Could you check a few things on this model? Use its own coordinates, in mm. A direction names the side the tool comes from. Give positions to 0.01 mm unless a question says otherwise; leave off trailing zeros. Write each loop counter-clockwise with the first axis right and the second up, starting at its lowest first coordinate (ties: lowest second). Pieces come first, ordered by that corner, then holes. Notation, with made-up numbers: M 59.5,16 L 107.5,16 A30 cw 107.5,53 Z; hole C -38.75,64.5 d5. An arc over 180 degrees is marked long. Write each question's results on one line, items separated by ' | '. Start each with the question number.
from build123d import *

# Parameters (mm, degrees)
S_CYL1_R        = 19
BOSS_1_DEPTH    = 7
BOSS_2_DEPTH    = 2.1
S_BOX3_W        = 28.2
S_BOX3_H        = 10
BOSS_3_DEPTH    = 1.5
S_BOX4_W        = 37.6
S_BOX4_H        = 47
BOSS_4_DEPTH    = 14.2
BOSS_5_DEPTH    = 23
BOSS_6_DEPTH    = 22
S_BOX7_W        = 36.1
S_BOX7_H        = 3
BOSS_7_DEPTH    = 31.8
S_BOX8_W        = 36.1
S_BOX8_H        = 3
BOSS_8_DEPTH    = 31.8
S_BOX9_W        = 36.1
S_BOX9_H        = 52.4
BOSS_9_DEPTH    = 3
S_BOX10_W       = 36.1
S_BOX10_H       = 52.4
BOSS_10_DEPTH   = 3
S_BOX11_W       = 4.6
S_BOX11_H       = 52.4
BOSS_11_DEPTH   = 31.8
S_HOLE12_R      = 10.5
HOLE_12_DEPTH   = 4.8
S_CUT13_W       = 4.75
S_CUT13_H       = 19.5
POCKET_13_DEPTH = 19.4
S_CUT14_W       = 4.75
S_CUT14_H       = 8.8
POCKET_14_DEPTH = 16.4
S_CUT15_W       = 4.75
S_CUT15_H       = 11
POCKET_15_DEPTH = 7
S_CUT16_W       = 2.9
S_CUT16_H       = 20
POCKET_16_DEPTH = 16.4
S_HOLE17_R      = 1.1
HOLE_17_DEPTH   = 4.8
S_HOLE18_R      = 2.3
HOLE_18_DEPTH   = 1.7
S_HOLE19_R      = 1.1
HOLE_19_DEPTH   = 4.8
S_HOLE20_R      = 2.3
HOLE_20_DEPTH   = 1.7
S_HOLE21_R      = 1.1
HOLE_21_DEPTH   = 4.8
S_HOLE22_R      = 2.3
HOLE_22_DEPTH   = 1.7
CUT_23_DEPTH    = 6.1
S_HOLE24_R      = 3.5
HOLE_24_DEPTH   = 10.6
S_HOLE25_R      = 1.7
HOLE_25_DEPTH   = 10.6
S_HOLE26_R      = 1.7
HOLE_26_DEPTH   = 10.6
S_HOLE27_R      = 1.7
HOLE_27_DEPTH   = 10.6
S_HOLE28_R      = 1.7
HOLE_28_DEPTH   = 10.6
S_HOLE29_R      = 3.2
HOLE_29_DEPTH   = 7.6
S_HOLE30_R      = 3.2
HOLE_30_DEPTH   = 7.6
S_HOLE31_R      = 3.2
HOLE_31_DEPTH   = 7.6
S_HOLE32_R      = 3.2
HOLE_32_DEPTH   = 7.6


with BuildPart() as part:
    # S_cyl1 → Boss_1 (new body)
    with BuildSketch(Plane.XY.offset(23)):
        Circle(S_CYL1_R)
    extrude(amount=BOSS_1_DEPTH)

    # S_prism2 → Boss_2 (add)
    with BuildSketch(Plane.XY.offset(21)):
        with BuildLine():
            Line((-15.491933385, -11), (15.491933385, -11))
            ThreePointArc((15.491933385, -11), (19, 0), (15.491933385, 11))
            Line((15.491933385, 11), (-15.491933385, 11))
            ThreePointArc((-15.491933385, 11), (-19, 0), (-15.491933385, -11))
        make_face()
    extrude(amount=BOSS_2_DEPTH)

    # S_box3 → Boss_3 (add)
    with BuildSketch(Plane.XY.offset(19.6)):
        with Locations((-0.1, 0)):
            Rectangle(S_BOX3_W, S_BOX3_H)
    extrude(amount=BOSS_3_DEPTH)

    # S_box4 → Boss_4 (add)
    with BuildSketch(Plane.XY.offset(15.8)):
        with Locations((-35.2, -11.5)):
            Rectangle(S_BOX4_W, S_BOX4_H)
    extrude(amount=BOSS_4_DEPTH)

    # S_prism5 → Boss_5 (add)
    with BuildSketch(Plane(origin=(-11.5, 0, 0), x_dir=(0, 0, -1), z_dir=(1, 0, 0))):
        Polygon((-21.05, -11), (-21.05, 12), (-23.1, 15), (-23.1, -12.5), align=None)
    extrude(amount=BOSS_5_DEPTH)

    # S_prism6 → Boss_6 (add)
    with BuildSketch(Plane(origin=(0, -11, 0), x_dir=(1, 0, 0), z_dir=(0, 1, 0))):
        Polygon((-16.45, -21.1), (-16.45, -19.9), (-14.8, -21.1), align=None)
    extrude(amount=BOSS_6_DEPTH)

    # S_box8 → Boss_8 (add)
    with BuildSketch(Plane.XY.offset(-15.9)):
        with Locations((-36.85, 12.2)):
            Rectangle(S_BOX8_W, S_BOX8_H)
    extrude(amount=BOSS_8_DEPTH)



with BuildPart() as body_2:
    # S_box7 → Boss_7 (new body)
    with BuildSketch(Plane.XY.offset(-15.9)):
        with Locations((-36.85, -37.2)):
            Rectangle(S_BOX7_W, S_BOX7_H)
    extrude(amount=BOSS_7_DEPTH)


with BuildPart() as part_1:
    add(part.part)

    add(body_2.part)  # Boss_9 merges body 2
    # S_box9 → Boss_9 (add)
    with BuildSketch(Plane.XY.offset(-15.9)):
        with Locations((-36.85, -12.5)):
            Rectangle(S_BOX9_W, S_BOX9_H)
    extrude(amount=BOSS_9_DEPTH)

    # S_box10 → Boss_10 (add)
    with BuildSketch(Plane.XY.offset(12.9)):
        with Locations((-36.85, -12.5)):
            Rectangle(S_BOX10_W, S_BOX10_H)
    extrude(amount=BOSS_10_DEPTH)

    # S_box11 → Boss_11 (add)
    with BuildSketch(Plane.XY.offset(-15.9)):
        with Locations((-52.6, -12.5)):
            Rectangle(S_BOX11_W, S_BOX11_H)
    extrude(amount=BOSS_11_DEPTH)

    # S_hole12 → Hole_12 (cut)
    with BuildSketch(Plane(origin=(-55, 0, 0), x_dir=(0, 0, -1), z_dir=(1, 0, 0))):
        with Locations(Location((0, 0, 0), (0, 0, 180))):
            Circle(S_HOLE12_R)
    extrude(amount=HOLE_12_DEPTH, mode=Mode.SUBTRACT)

    # S_cut13 → Pocket_13 (cut)
    with BuildSketch(Plane.XY.offset(-9.7)):
        with Locations((-52.625, -20.65)):
            Rectangle(S_CUT13_W, S_CUT13_H)
    extrude(amount=POCKET_13_DEPTH, mode=Mode.SUBTRACT)

    # S_cut14 → Pocket_14 (cut)
    with BuildSketch(Plane.XY.offset(-8.2)):
        with Locations((-52.625, -34.8)):
            Rectangle(S_CUT14_W, S_CUT14_H)
    extrude(amount=POCKET_14_DEPTH, mode=Mode.SUBTRACT)

    # S_cut15 → Pocket_15 (cut)
    with BuildSketch(Plane.XY.offset(-3.5)):
        with Locations((-52.625, -5.5)):
            Rectangle(S_CUT15_W, S_CUT15_H)
    extrude(amount=POCKET_15_DEPTH, mode=Mode.SUBTRACT)

    # S_cut16 → Pocket_16 (cut)
    with BuildSketch(Plane.XY.offset(-16.4)):
        with Locations((-53.65, 0)):
            Rectangle(S_CUT16_W, S_CUT16_H)
    extrude(amount=POCKET_16_DEPTH, mode=Mode.SUBTRACT)

    # S_hole17 → Hole_17 (cut)
    with BuildSketch(Plane(origin=(-55, 0, 0), x_dir=(0, 0, -1), z_dir=(1, 0, 0))):
        with Locations(Location((-10.25, -8.3, 0), (0, 0, 180))):
            Circle(S_HOLE17_R)
    extrude(amount=HOLE_17_DEPTH, mode=Mode.SUBTRACT)

    # S_hole18 → Hole_18 (cut)
    with BuildSketch(Plane(origin=(-55, 0, 0), x_dir=(0, 0, -1), z_dir=(1, 0, 0))):
        with Locations((-10.25, -8.3)):
            Circle(S_HOLE18_R)
    extrude(amount=HOLE_18_DEPTH, mode=Mode.SUBTRACT)

    # S_hole19 → Hole_19 (cut)
    with BuildSketch(Plane(origin=(-55, 0, 0), x_dir=(0, 0, -1), z_dir=(1, 0, 0))):
        with Locations(Location((10.25, -32.75, 0), (0, 0, 180))):
            Circle(S_HOLE19_R)
    extrude(amount=HOLE_19_DEPTH, mode=Mode.SUBTRACT)

    # S_hole20 → Hole_20 (cut)
    with BuildSketch(Plane(origin=(-55, 0, 0), x_dir=(0, 0, -1), z_dir=(1, 0, 0))):
        with Locations((10.25, -32.75)):
            Circle(S_HOLE20_R)
    extrude(amount=HOLE_20_DEPTH, mode=Mode.SUBTRACT)

    # S_hole21 → Hole_21 (cut)
    with BuildSketch(Plane(origin=(-55, 0, 0), x_dir=(0, 0, -1), z_dir=(1, 0, 0))):
        with Locations(Location((-10.25, -32.75, 0), (0, 0, 180))):
            Circle(S_HOLE21_R)
    extrude(amount=HOLE_21_DEPTH, mode=Mode.SUBTRACT)

    # S_hole22 → Hole_22 (cut)
    with BuildSketch(Plane(origin=(-55, 0, 0), x_dir=(0, 0, -1), z_dir=(1, 0, 0))):
        with Locations((-10.25, -32.75)):
            Circle(S_HOLE22_R)
    extrude(amount=HOLE_22_DEPTH, mode=Mode.SUBTRACT)

    # S_pcut23 → Cut_23 (cut)
    with BuildSketch(Plane.XY.offset(20.9)):
        with BuildLine():
            Line((-14.792307772, 12.858756968), (-11.547056577, 10.037703144))
            ThreePointArc((-11.547056577, 10.037703144), (11.72047998, 9.834650428), (7.880082546, -13.114659701))
            Line((7.880082546, -13.114659701), (10.094746268, -16.800479094))
            ThreePointArc((10.094746268, -16.800479094), (15.014471085, 12.59863715), (-14.792307772, 12.858756968))
        make_face()
    extrude(amount=CUT_23_DEPTH, mode=Mode.SUBTRACT)

    # S_hole24 → Hole_24 (cut)
    with BuildSketch(Plane.XY.offset(19.5)):
        Circle(S_HOLE24_R)
    extrude(amount=HOLE_24_DEPTH, mode=Mode.SUBTRACT)

    # S_hole25 → Hole_25 (cut)
    with BuildSketch(Plane.XY.offset(19.5)):
        with Locations((7, 0)):
            Circle(S_HOLE25_R)
    extrude(amount=HOLE_25_DEPTH, mode=Mode.SUBTRACT)

    # S_hole26 → Hole_26 (cut)
    with BuildSketch(Plane.XY.offset(19.5)):
        with Locations((0, 7)):
            Circle(S_HOLE26_R)
    extrude(amount=HOLE_26_DEPTH, mode=Mode.SUBTRACT)

    # S_hole27 → Hole_27 (cut)
    with BuildSketch(Plane.XY.offset(19.5)):
        with Locations((-7, 0)):
            Circle(S_HOLE27_R)
    extrude(amount=HOLE_27_DEPTH, mode=Mode.SUBTRACT)

    # S_hole28 → Hole_28 (cut)
    with BuildSketch(Plane.XY.offset(19.5)):
        with Locations((0, -7)):
            Circle(S_HOLE28_R)
    extrude(amount=HOLE_28_DEPTH, mode=Mode.SUBTRACT)

    # S_hole29 → Hole_29 (cut)
    with BuildSketch(Plane.XY.offset(19.4)):
        with Locations(Location((7, 0, 0), (0, 0, 180))):
            Circle(S_HOLE29_R)
    extrude(amount=HOLE_29_DEPTH, mode=Mode.SUBTRACT)

    # S_hole30 → Hole_30 (cut)
    with BuildSketch(Plane.XY.offset(19.4)):
        with Locations(Location((0, 7, 0), (0, 0, 218.682187453))):
            Circle(S_HOLE30_R)
    extrude(amount=HOLE_30_DEPTH, mode=Mode.SUBTRACT)

    # S_hole31 → Hole_31 (cut)
    with BuildSketch(Plane.XY.offset(19.4)):
        with Locations(Location((-7, 0, 0), (0, 0, 180))):
            Circle(S_HOLE31_R)
    extrude(amount=HOLE_31_DEPTH, mode=Mode.SUBTRACT)

    # S_hole32 → Hole_32 (cut)
    with BuildSketch(Plane.XY.offset(19.4)):
        with Locations(Location((0, -7, 0), (0, 0, 141.317812547))):
            Circle(S_HOLE32_R)
    extrude(amount=HOLE_32_DEPTH, mode=Mode.SUBTRACT)


solid = part_1.part
Q1. If we section it at C-C (x = 0): Count the separate pieces of the cut face and the enclosed holes in it, plus the area to 3 significant figures.
Q2. If we mould it in two halves opening along X, with no side actions, what happens to faces 6 (the face through (-50.25, -37, 0)), 7 (the face through (-37, -38.7, 0)), 8 (the face through (-14, 11, 22))? For each: pulls with the +X half, pulls with the -X half, needs draft (parallel to the pull), parting line crosses it, or undercut.
Q3. For faces 1 (the face through (4.044, 1.226, 23.248)), 2 (the face through (-54, 10, -10)), 3 (the face through (-53.3, -34, -11)), 4 (the face through (-53, -34, 8.2)), 5 (the face through (-53, -21, -9.7)), which set-ups out of +Z, -Z, +X, -X, +Y, -Y let a thin tool reach every point of the face, with its end or its side?
Q4. If we section it at B-B (y = -32.75): Please give me the cut outline in (x, z), plus the area to 3 significant figures.
Q5. Please list where these lines run through material, in increasing order: line 1 (Y direction, x = 0, z = 29); line 2 (Z direction, x = -26, y = -17.5); line 3 (Y direction, x = -37, z = 12). Write a range as [from, to].
Q6. If we section it at A-A (z = 0): Please give me the cut outline in (x, y).
Q7. I'm going to push flat-ended pins straight in: P1, Ø4, axis at x = -23, z = -8.5, coming from the +Y side; P2, Ø8.5, axis at x = -7, y = 0, coming from the +Z side; P3, Ø1.4, axis at y = -7.5, z = 9.5, coming from the -X side; P4, Ø7, axis at y = -12, z = 21, coming from the -X side. Where does each tip first touch, or does it pass through?
Q8. If we section it at D-D (z = 26): Please give me the cut outline in (x, y), plus the area to 3 significant figures.
Determined:
1) separate pieces: 4 | enclosed holes: 0 | area: 142 mm²
2) face 6: pulls with the -X half | face 7: needs draft | face 8: undercut
3) face 1: -Z | face 2: -Z, -X | face 3: -X | face 4: -X, -Y | face 5: +X, -X
4) outline: M -54.9,-15.9 L -18.8,-15.9 L -18.8,-12.9 L -50.3,-12.9 L -50.3,-11.35 L -53.3,-11.35 L -53.3,-12.55 L -54.9,-12.55 Z; M -54.9,12.55 L -53.3,12.55 L -53.3,11.35 L -50.3,11.35 L -50.3,12.9 L -18.8,12.9 L -18.8,15.8 L -16.4,15.8 L -16.4,30 L -54,30 L -54,15.9 L -54.9,15.9 Z; M -53.3,-9.15 L -50.3,-9.15 L -50.3,-8.2 L -53.3,-8.2 Z; M -53.3,8.2 L -50.3,8.2 L -50.3,9.15 L -53.3,9.15 Z | area: 763 mm²
5) line 1: y = [-19, -8.7], [-5.3, -3.5], [3.5, 5.3], [8.7, 19] | line 2: z = [-15.9, -12.9], [12.9, 30] | line 3: y = [-38.7, -35.7], [10.7, 13.7]
6) outline: M -54.9,10.5 L -50.3,10.5 L -50.3,10.7 L -18.8,10.7 L -18.8,13.7 L -54.9,13.7 Z; M -50.25,-38.7 L -18.8,-38.7 L -18.8,-35.7 L -50.25,-35.7 Z
7) P1: stops at y = 13.7 | P2: stops at z = 30 | P3: stops at x = -53.3 | P4: stops at x = -54
8) outline: M -54,-35 L -16.4,-35 L -16.4,-9.59 A19 ccw 9.79,-16.29 L 7.88,-13.11 A15.3 ccw long -11.55,10.04 L -14.34,12.47 A19 ccw -16.4,9.59 L -16.4,12 L -54,12 Z; hole C -7,0 d6.4; hole C 0,0 d7; hole C 0,-7 d6.4; hole C 0,7 d6.4; hole C 7,0 d6.4 | area: 2,480 mm²
